Read the model definition and answer for the solid it produces. Units are mm, in the model's axes. Coordinates: 2 decimals unless noted, no trailing zeros. Loops run counter-clockwise (first coordinate to the right, second up) from the corner with the lowest first, then second, coordinate; pieces in that order, holes last. Notation, with made-up numbers: (85.5, -16) - (133.5, -16) arc R9 ccw to (133.5, -1) - close; hole circle Ø2 at (42.25, 77). An arc over 180 degrees is marked (long way). Use CSV: the item, a comma, the result in double quotes.
```python
from build123d import *

# Parameters (mm, degrees)
BOSS_EXTRUDE1_DEPTH  = 4.7625
M4_CLEARANCE_HOLE1_D = 4.5
SKETCH4_R            = 6.35
SKETCH4_R_2          = 9.5
CUT_EXTRUDE1_DEPTH   = 85.681745462


with BuildPart() as part:
    # Sketch1 → Boss-Extrude1 (new body)
    with BuildSketch(Plane.XY):
        with BuildLine():
            ThreePointArc((68.668145751, 29.139971157), (66.93396374, 26.544584367), (66.325, 23.483116908))
            Line((66.325, 23.483116908), (66.325, -23.483116908))
            ThreePointArc((66.325, -23.483116908), (66.93396374, -26.544584367), (68.668145751, -29.139971157))
            Line((68.668145751, -29.139971157), (70.973014298, -31.444839705))
            ThreePointArc((70.973014298, -31.444839705), (71.257349949, -38.916180607), (63.829230118, -39.767542704))
            Line((63.829230118, -39.767542704), (60.979833165, -36.918145751))
            ThreePointArc((60.979833165, -36.918145751), (58.384446374, -35.18396374), (55.322978915, -34.575))
            Line((55.322978915, -34.575), (12.648995245, -34.575))
            ThreePointArc((12.648995245, -34.575), (8.086292992, -36.003717922), (5.153294359, -39.779562963))
            ThreePointArc((5.153294359, -39.779562963), (0, -43.3577), (-5.153294359, -39.779562963))
            ThreePointArc((-5.153294359, -39.779562963), (-8.086292992, -36.003717922), (-12.648995245, -34.575))
            Line((-12.648995245, -34.575), (-55.322978915, -34.575))
            ThreePointArc((-55.322978915, -34.575), (-58.384446374, -35.18396374), (-60.979833165, -36.918145751))
            Line((-60.979833165, -36.918145751), (-63.829230118, -39.767542704))
            ThreePointArc((-63.829230118, -39.767542704), (-71.257349949, -38.916180607), (-70.973014298, -31.444839705))
            Line((-70.973014298, -31.444839705), (-68.668145751, -29.139971157))
            ThreePointArc((-68.668145751, -29.139971157), (-66.93396374, -26.544584367), (-66.325, -23.483116908))
            Line((-66.325, -23.483116908), (-66.325, 23.483116908))
            ThreePointArc((-66.325, 23.483116908), (-66.93396374, 26.544584367), (-68.668145751, 29.139971157))
            Line((-68.668145751, 29.139971157), (-70.973014298, 31.444839705))
            ThreePointArc((-70.973014298, 31.444839705), (-71.257349949, 38.916180607), (-63.829230118, 39.767542704))
            Line((-63.829230118, 39.767542704), (-60.979833165, 36.918145751))
            ThreePointArc((-60.979833165, 36.918145751), (-58.384446374, 35.18396374), (-55.322978915, 34.575))
            Line((-55.322978915, 34.575), (-12.648995245, 34.575))
            ThreePointArc((-12.648995245, 34.575), (-8.086292992, 36.003717922), (-5.153294359, 39.779562963))
            ThreePointArc((-5.153294359, 39.779562963), (0, 43.3577), (5.153294359, 39.779562963))
            ThreePointArc((5.153294359, 39.779562963), (8.086292992, 36.003717922), (12.648995245, 34.575))
            Line((12.648995245, 34.575), (55.322978915, 34.575))
            ThreePointArc((55.322978915, 34.575), (58.384446374, 35.18396374), (60.979833165, 36.918145751))
            Line((60.979833165, 36.918145751), (63.829230118, 39.767542704))
            ThreePointArc((63.829230118, 39.767542704), (71.257349949, 38.916180607), (70.973014298, 31.444839705))
            Line((70.973014298, 31.444839705), (68.668145751, 29.139971157))
        make_face()
    extrude(amount=-BOSS_EXTRUDE1_DEPTH)

    # M4 Clearance Hole1 (through all)
    with Locations(Plane(origin=(0, 0, -4.7625), x_dir=(-1, 0, 0), z_dir=(0, 0, -1))):
        with Locations((-67.083927001, -35.333927001), (-67.083927001, 35.333927001), (0, 37.8577), (67.083927001, 35.333927001), (67.083927001, -35.333927001), (0, -37.8577)):
            Hole(M4_CLEARANCE_HOLE1_D / 2)

    # Sketch4 → Cut-Extrude1 (cut, through all)
    with BuildSketch(Plane(origin=(0, 0, -4.7625), x_dir=(-1, 0, 0), z_dir=(0, 0, -1))):
        Circle(SKETCH4_R)
        with Locations((-23.8125, 0)):
            Circle(SKETCH4_R_2)
        with Locations((23.8125, 0)):
            Circle(SKETCH4_R_2)
    extrude(amount=-CUT_EXTRUDE1_DEPTH, mode=Mode.SUBTRACT)


solid = part.part
```
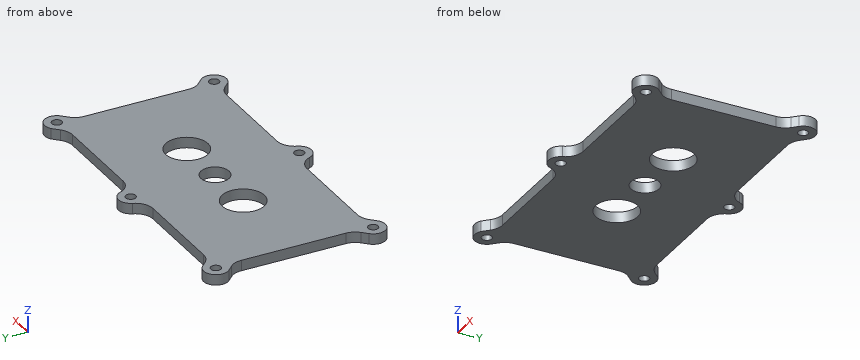
Q1. Given P1, Ø1.4, axis at y = 2.5, z = -3.5, coming from the -X side (3 decimals); P2, Ø2.5, axis at x = 30.5, z = -2, coming from the -Y side (3 decimals); P3, Ø2.5, axis at y = -7.5, z = -3, coming from the +X side (3 decimals), each flat-ended and moving along its own axis, determine where each tip first touches the part or whether it passes through.
Reported:
P1,"stops at x = -66.325"
P2,"stops at y = -34.575"
P3,"stops at x = 66.325"
Q2. The part is cut by section C-C on x = 17. Determine the outline of the cut face in (y, z) (1 decimal).
Reported:
outline,"(-34.6, -4.8) - (-6.6, -4.8) - (-6.6, 0) - (-34.6, 0) - close; (6.6, -4.8) - (34.6, -4.8) - (34.6, 0) - (6.6, 0) - close"
Q3. The part is cut by section A-A on y = 0. Give the number of separate pieces and of enclosed holes in the cut face, and give its area (3 significant figures).
Reported:
separate pieces,"4"
enclosed holes,"0"
area,"390 mm²"
Q4. Find the intervals of material crossed by probe 1 along X at (y, z) = (0.5, -4.3) (3 decimals); probe 2 along X at (y, z) = (2, -0.35) (3 decimals); probe 3 along X at (y, z) = (6.5, -0.25) (3 decimals), in increasing order. Write a range as [from, to].
Reported:
probe 1,"x = [-66.325, -33.299], [-14.326, -6.33], [6.33, 14.326], [33.299, 66.325]"
probe 2,"x = [-66.325, -33.1], [-14.525, -6.027], [6.027, 14.525], [33.1, 66.325]"
probe 3,"x = [-66.325, -30.741], [-16.884, 16.884], [30.741, 66.325]"
Q5. The part is cut by section D-D on x = -19. Determine the outline of the cut face in (y, z) (1 decimal), and give its area (3 significant figures).
Reported:
outline,"(-34.6, -4.8) - (-8.2, -4.8) - (-8.2, 0) - (-34.6, 0) - close; (8.2, -4.8) - (34.6, -4.8) - (34.6, 0) - (8.2, 0) - close"
area,"251 mm²"
Q6. The part is cut by section B-B on x = 0. Determine the outline of the cut face in (y, z), and give its area (3 significant figures).
Reported:
outline,"(-43.36, -4.76) - (-40.11, -4.76) - (-40.11, 0) - (-43.36, 0) - close; (-35.61, -4.76) - (-6.35, -4.76) - (-6.35, 0) - (-35.61, 0) - close; (6.35, -4.76) - (35.61, -4.76) - (35.61, 0) - (6.35, 0) - close; (40.11, -4.76) - (43.36, -4.76) - (43.36, 0) - (40.11, 0) - close"
area,"310 mm²"
